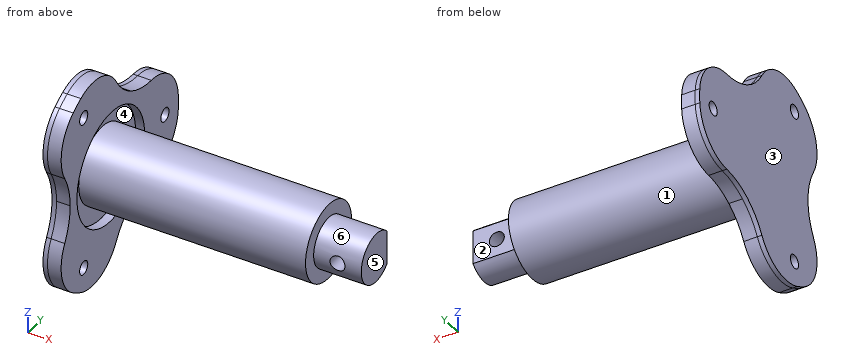
```python
from build123d import *

# Parameters (mm, degrees)
SKETCH_1_R               = 25
EXTRUDE_1_DEPTH          = 3
CUT_EXTRUDE_START        = -3
CUT_EXTRUDE_1_DEPTH      = 3
PATTERN_CIRCULAR_1_COUNT = 3
FILLET_1_R               = 10
SKETCH_3_R               = 8.5
EXTRUDE_2_DEPTH          = 48
SKETCH_5_R               = 1.5
CUT_EXTRUDE_2_DEPTH      = 52
PATTERN_CIRCULAR_2_COUNT = 3
SKETCH_7_R               = 5.5
EXTRUDE_3_DEPTH          = 10.5
SKETCH_8_W               = 10.294353596
SKETCH_8_H               = 3.679030571
CUT_EXTRUDE_3_DEPTH      = 10.5
CUT_EXTRUDE_START_2      = -2
SKETCH_12_R              = 12.5
SKETCH_12_R_2            = 8.5
CUT_EXTRUDE_6_DEPTH      = 2
EXTRUDE_START            = 1
SKETCH_13_R              = 1.5
EXTRUDE_4_DEPTH          = 1
HOLE_WIZARD_M4_1_D       = 3.3


with BuildPart() as part:
    # 草图1 → 凸台-拉伸1 (new body)
    with BuildSketch(Plane(origin=(0, 0, 0), x_dir=(0, 0, -1), z_dir=(1, 0, 0))):
        Circle(SKETCH_1_R)
    extrude(amount=EXTRUDE_1_DEPTH)

    # 草图2 → 切除-拉伸1 (cut)
    with BuildSketch(Plane(origin=(3, 0, 0), x_dir=(0, 0, -1), z_dir=(1, 0, 0)).offset(CUT_EXTRUDE_START)):
        with BuildLine():
            ThreePointArc((24.999979393, 0.032098836), (24.143986785, 6.485977345), (21.650635095, 12.5))
            Line((21.650635095, 12.5), (12.990381057, 7.5))
            ThreePointArc((12.990381057, 7.5), (18.059856782, 2.261897365), (24.999979393, 0.032098836))
        make_face()
        with BuildLine():
            ThreePointArc((12.527788104, 21.634567831), (17.689014542, 17.666317232), (21.650635095, 12.5))
            ThreePointArc((21.650635095, 12.5), (24.143986785, 6.485977345), (24.999979393, 0.032098836))
            ThreePointArc((24.999979393, 0.032098836), (36.234743272, 4.052129412), (40.980762114, 15))
            ThreePointArc((40.980762114, 15), (29.387034993, 29.608124625), (12.527788104, 21.634567831))
        make_face()
        with BuildLine():
            Line((12.990381057, 7.5), (21.650635095, 12.5))
            ThreePointArc((21.650635095, 12.5), (17.689014542, 17.666317232), (12.527788104, 21.634567831))
            ThreePointArc((12.527788104, 21.634567831), (10.98878897, 14.509346079), (12.990381057, 7.5))
        make_face()
    cut_extrude_1 = extrude(amount=CUT_EXTRUDE_1_DEPTH, mode=Mode.SUBTRACT)

    # 阵列(圆周)1: 切除-拉伸1 ×3 about axis
    pattern_circular_1_axis = Axis((0, 0, 0), (1, 0, 0))
    for i in range(1, PATTERN_CIRCULAR_1_COUNT):
        add(cut_extrude_1.rotate(pattern_circular_1_axis, i * 360 / PATTERN_CIRCULAR_1_COUNT), mode=Mode.SUBTRACT)

    # 圆角1
    fillet_1_edges = [part.edges().sort_by_distance(p)[0] for p in [
        (1.5, 0.032098836, 24.999979393),
        (1.5, 21.634567831, 12.527788104),
        (1.5, -21.666666667, -12.472191289),
        (1.5, -21.666666667, 12.472191289),
        (1.5, 21.634567831, -12.527788104),
        (1.5, 0.032098836, -24.999979393),
    ]]
    fillet(fillet_1_edges, radius=FILLET_1_R)

    # 草图3 → 凸台-拉伸2 (add)
    with BuildSketch(Plane(origin=(3, 0, 0), x_dir=(0, 0, -1), z_dir=(1, 0, 0))):
        Circle(SKETCH_3_R)
    extrude(amount=EXTRUDE_2_DEPTH)

    # 草图5 → 切除-拉伸2 (cut)
    with BuildSketch(Plane.ZY):
        with Locations((0, 20)):
            Circle(SKETCH_5_R)
    cut_extrude_2 = extrude(amount=-CUT_EXTRUDE_2_DEPTH, mode=Mode.SUBTRACT)

    # 阵列(圆周)2: 切除-拉伸2 ×3 about axis
    pattern_circular_2_axis = Axis((0, 0, 0), (1, 0, 0))
    for i in range(1, PATTERN_CIRCULAR_2_COUNT):
        add(cut_extrude_2.rotate(pattern_circular_2_axis, i * 360 / PATTERN_CIRCULAR_2_COUNT), mode=Mode.SUBTRACT)

    # 草图7 → 凸台-拉伸3 (add)
    with BuildSketch(Plane(origin=(51, 0, 0), x_dir=(0, 0, -1), z_dir=(1, 0, 0))):
        with Locations(Location((0, 0, 0), (0, 0, 180))):
            Circle(SKETCH_7_R)
    extrude(amount=EXTRUDE_3_DEPTH)

    # 草图8 → 切除-拉伸3 (cut)
    with BuildSketch(Plane(origin=(61.5, 0, 0), x_dir=(0, 0, -1), z_dir=(1, 0, 0))):
        with Locations((0, 5.839515286)):
            Rectangle(SKETCH_8_W, SKETCH_8_H)
    extrude(amount=-CUT_EXTRUDE_3_DEPTH, mode=Mode.SUBTRACT)

    # 草图12 → 切除-拉伸6 (cut)
    with BuildSketch(Plane(origin=(3, 0, 0), x_dir=(0, 0, -1), z_dir=(1, 0, 0)).offset(CUT_EXTRUDE_START_2)):
        Circle(SKETCH_12_R)
        Circle(SKETCH_12_R_2, mode=Mode.SUBTRACT)
    extrude(amount=CUT_EXTRUDE_6_DEPTH, mode=Mode.SUBTRACT)

    # 草图13 → 凸台-拉伸4 (add)
    with BuildSketch(Plane.ZY.offset(EXTRUDE_START)):
        with BuildLine():
            ThreePointArc((-18.464089251, 2.019259302), (-12.990381057, 7.5), (-10.980774478, 14.980740698))
            ThreePointArc((-10.980774478, 14.980740698), (-8.274973062, 21.808572714), (-1.634637867, 24.94650194))
            ThreePointArc((-1.634637867, 24.94650194), (0, 25), (1.634637867, 24.94650194))
            ThreePointArc((1.634637867, 24.94650194), (8.274973062, 21.808572714), (10.980774478, 14.980740698))
            ThreePointArc((10.980774478, 14.980740698), (12.990381057, 7.5), (18.464089251, 2.019259302))
            ThreePointArc((18.464089251, 2.019259302), (23.024264522, -3.737949469), (22.421623349, -11.057613051))
            ThreePointArc((22.421623349, -11.057613051), (21.650635095, -12.5), (20.786985482, -13.888888889))
            ThreePointArc((20.786985482, -13.888888889), (14.749291459, -18.070623245), (7.483314774, -17))
            ThreePointArc((7.483314774, -17), (0, -15), (-7.483314774, -17))
            ThreePointArc((-7.483314774, -17), (-14.749291459, -18.070623245), (-20.786985482, -13.888888889))
            ThreePointArc((-20.786985482, -13.888888889), (-21.650635095, -12.5), (-22.421623349, -11.057613051))
            ThreePointArc((-22.421623349, -11.057613051), (-23.024264522, -3.737949469), (-18.464089251, 2.019259302))
        make_face()
        with Locations((0, 20)):
            Circle(SKETCH_13_R, mode=Mode.SUBTRACT)
        with Locations((-17.320508076, -10)):
            Circle(SKETCH_13_R, mode=Mode.SUBTRACT)
        with Locations((17.320508076, -10)):
            Circle(SKETCH_13_R, mode=Mode.SUBTRACT)
    extrude(amount=-EXTRUDE_4_DEPTH)

    # M4 螺纹孔1 (through all)
    with Locations(Plane(origin=(0, 4, 0), x_dir=(1, 0, 0), z_dir=(0, 1, 0))):
        with Locations((56.25, 0)):
            Hole(HOLE_WIZARD_M4_1_D / 2)


solid = part.part
```
Work out the finished part from the listing and answer in its coordinate system (mm). Face numbers are marked on the shaded views. A direction names the side the tool comes from. Give positions to 0.01 mm unless a question says otherwise; leave off trailing zeros. Loops run counter-clockwise (first coordinate to the right, second up) from the corner with the lowest first, then second, coordinate; pieces in that order, holes last. Notation, with made-up numbers: (27, 29) -> (47, 29) arc R7 ccw to (47, 39) -> close; hole circle Ø7 at (-1.5, 23.25). An arc over 180 degrees is marked (long way). One line per question, with ' | ' between items. Start each with the question number.
1) Section C-C, the plane x = 11 is taken. Determine the outline of the cut face in (y, z), then the cut area to 3 significant figures.
2) Determine the mould class of the marked faces 4, 5 and 6 for opening direction Z: +Z half, -Z half, draft (parallel to the pull), parting line (faces both ways), or undercut.
3) For the marked faces 1, 2 and 3, determine the directions among +Z, -Z, +X, -X, +Y, -Y from which every point of the face is accessible in a straight line to the end or side of a thin tool.
4) Section A-A, the plane x = 56.25 is taken. Determine the outline of the cut face in (y, z), then the cut area to 3 significant figures.
5) Section B-B, the plane y = 5.5 is taken. Determine the outline of the cut face in (x, z).
6) Each of these flat-tipped pins is pushed along its axis until it touches: pin 1 (6 mm diameter, centred on x = 30, z = 6, fed in from +Y); pin 2 (10 mm diameter, centred on x = 24.5, z = 2.5, fed in from +Y); pin 3 (8 mm diameter, centred on x = 39, y = 0, fed in from +Z); pin 4 (3.5 mm diameter, centred on y = -10, z = 17.32, fed in from -X). Where does it stop, or does it pass through?
7) Straight lines are drawn through the part: L1, parallel to Z at x = 0, y = -10; L2, parallel to Z at x = 1.55, y = -10; L3, parallel to Z at x = 27, y = 4. For each, find the intervals that lie inside material, in ascending order.
Resolved:
1) outline: circle Ø17 at (0, 0) | area: 227 mm2
2) face 4: undercut | face 5: draft | face 6: parting line
3) face 1: +X | face 2: +Z, -Z, +X, +Y | face 3: +Z, -Z, -X, +Y, -Y
4) outline: (-5.25, -1.65) arc R5.5 ccw to (4, -3.77) -> (4, -1.65) -> close; (-5.25, 1.65) -> (4, 1.65) -> (4, 3.77) arc R5.5 ccw to start | area: 56.2 mm2
5) outline: (-1, -14.37) -> (3, -14.37) -> (3, -11.22) -> (1, -11.22) -> (1, -6.48) -> (51, -6.48) -> (51, 6.48) -> (1, 6.48) -> (1, 11.22) -> (3, 11.22) -> (3, 14.37) -> (-1, 14.37) -> close
6) pin 1: y = 7.95 | pin 2: y = 8.5 | pin 3: z = 8.5 | pin 4: x = -1
7) L1: -22.87 to -18.82, -15.82 to 15.82, 18.82 to 22.87 | L2: -22.87 to -18.82, -15.82 to -7.5, 7.5 to 15.82, 18.82 to 22.87 | L3: -7.5 to 7.5
